```python
from build123d import *

# Parameters (mm, degrees)
F0_W     = 63.917339
F0_H     = 42.158244
F1_DEPTH = 50.8
F3_D     = 6.35
F4_R     = 5.08
F5_SIZE  = 5.08


with BuildPart() as f1:
    # F0 (on Front) → F1 (new body)
    with BuildSketch(Plane.XZ):
        with Locations((4.646473, 2.719886)):
            Rectangle(F0_W, F0_H)
    extrude(amount=F1_DEPTH)

    # F3 (through all)
    with Locations(Plane.XZ.offset(50.8)):
        with Locations((-15.938915, 12.444086)):
            Hole(F3_D / 2)

    # F4
    f4_edges = [f1.edges().sort_by_distance(p)[0] for p in [
        (36.605142, -25.4, 23.799008),
    ]]
    fillet(f4_edges, radius=F4_R)

    # F5
    f5_edges = [f1.edges().sort_by_distance(p)[0] for p in [
        (-27.312197, -25.4, 23.799008),
    ]]
    chamfer(f5_edges, length=F5_SIZE)


solid = f1.part
```
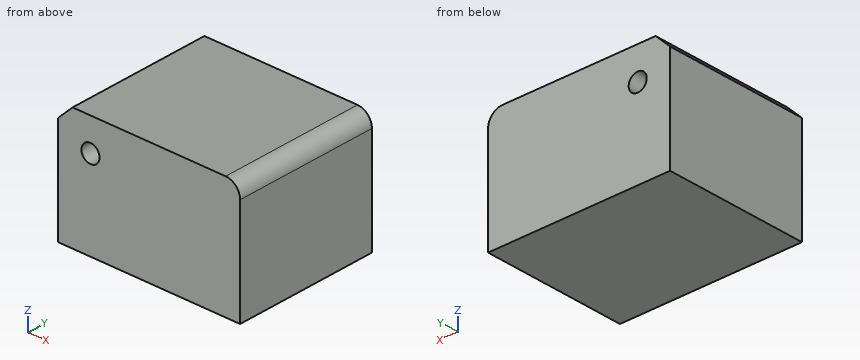
Model file for the job. Use its own axes, mm. Coordinates: 2 decimals unless noted, no trailing zeros. Write each loop counter-clockwise with the first axis right and the second up, starting at its lowest first coordinate (ties: lowest second). Pieces come first, ordered by that corner, then holes. Notation, with made-up numbers: (-19, 71) - (23, 71) arc R20 cw to (23, 79) - close; hole circle Ø8 at (-39, -28). An arc over 180 degrees is marked (long way). One line per item, written item: value. Start each with the question number.
1. Slice it at A-A (y = -25). Write the cut outline in (x, z) (3 decimals), plus the area to 3 significant figures.
2. Slice it at B-B (z = 21). Write the cut outline in (x, y), plus the area to 3 significant figures.
3. Flat gauge pin, fed straight in: pin 1 (10 mm diameter, centred on x = -16.5, z = -2, fed in from +Y). Where does the tip first touch, or does it go through?
4. Probe line 1 (X direction, y = -13, z = 15); line 2 (Z direction, x = 32, y = -17); line 3 (Z direction, x = -22.5, y = -45). List the from-to ranges inside material, lowest first. Write a range as from..to.
Answers below:
1. outline: (-27.312, -18.359) - (36.605, -18.359) - (36.605, 18.719) arc R5.08 ccw to (31.525, 23.799) - (-22.232, 23.799) - (-27.312, 18.719) - close; hole circle Ø6.35 at (-15.939, 12.444)
1. area: 2,640 mm^2
2. outline: (-25.03, -50.8) - (36.06, -50.8) - (36.06, 0) - (-25.03, 0) - close
2. area: 3,100 mm^2
3. pin 1: stops at y = 0
4. line 1: x = -27.31..-17.82, -14.06..36.61
4. line 2: z = -18.36..23.78
4. line 3: z = -18.36..23.53
